```python
from build123d import *

# Parameters (mm, degrees)
SKETCH_1_R          = 2
EXTRUDE_1_DEPTH     = 4
SKETCH_2_R          = 1.5
SKETCH_2_R_2        = 2
EXTRUDE_2_DEPTH     = 4
CUT_EXTRUDE_1_DEPTH = 174.943237868
FILLET_2_R          = 1
FILLET_3_R          = 1


with BuildPart() as part:
    # 草图1 → 凸台-拉伸1 (new body)
    with BuildSketch(Plane(origin=(0, 0, 0), x_dir=(1, 0, 0), z_dir=(0, 1, 0))):
        Polygon((0, 0), (0, -110), (-62.5, -110), (-62.5, -130), (97.5, -130), (97.5, -110), (35, -110), (35, 0), align=None)
        with Locations(Location((5, -5, 0), (0, 0, 270))):
            Circle(SKETCH_1_R, mode=Mode.SUBTRACT)
        with Locations(Location((30, -5, 0), (0, 0, 270))):
            Circle(SKETCH_1_R, mode=Mode.SUBTRACT)
        with Locations(Location((5, -35, 0), (0, 0, 270))):
            Circle(SKETCH_1_R, mode=Mode.SUBTRACT)
        with Locations(Location((30, -35, 0), (0, 0, 270))):
            Circle(SKETCH_1_R, mode=Mode.SUBTRACT)
        with Locations(Location((-52.5, -122.5, 0), (0, 0, 270))):
            Circle(SKETCH_1_R, mode=Mode.SUBTRACT)
        with Locations(Location((-32.5, -122.5, 0), (0, 0, 270))):
            Circle(SKETCH_1_R, mode=Mode.SUBTRACT)
        with Locations(Location((-12.5, -122.5, 0), (0, 0, 270))):
            Circle(SKETCH_1_R, mode=Mode.SUBTRACT)
        with Locations(Location((7.5, -122.5, 0), (0, 0, 270))):
            Circle(SKETCH_1_R, mode=Mode.SUBTRACT)
        with Locations(Location((27.5, -122.5, 0), (0, 0, 270))):
            Circle(SKETCH_1_R, mode=Mode.SUBTRACT)
        with Locations(Location((47.5, -122.5, 0), (0, 0, 270))):
            Circle(SKETCH_1_R, mode=Mode.SUBTRACT)
        with Locations(Location((67.5, -122.5, 0), (0, 0, 270))):
            Circle(SKETCH_1_R, mode=Mode.SUBTRACT)
        with Locations(Location((87.5, -122.5, 0), (0, 0, 270))):
            Circle(SKETCH_1_R, mode=Mode.SUBTRACT)
    extrude(amount=EXTRUDE_1_DEPTH)

    # 草图2 → 凸台-拉伸2 (add)
    # profile 1 of 2: a face of its own
    with BuildSketch(Plane(origin=(0, 4, 0), x_dir=(1, 0, 0), z_dir=(0, 1, 0))):
        Polygon((0, -40), (0, -53), (-26.149225941, -56.891259047), (-32, -65), (-32, -110), (-41, -110), (-41, -70.637206461), (-69.401796613, -110), (-62.5, -110), (-62.5, -130), (-80.5, -130), (-80.5, -110), (-33.599955214, -45), align=None)
        with Locations(Location((-35, -65, 0), (0, 0, 270))):
            Circle(SKETCH_2_R, mode=Mode.SUBTRACT)
        with Locations(Location((-35, -75, 0), (0, 0, 270))):
            Circle(SKETCH_2_R, mode=Mode.SUBTRACT)
        with Locations(Location((-72.5, -122.5, 0), (0, 0, 270))):
            Circle(SKETCH_2_R_2, mode=Mode.SUBTRACT)
    # profile 2 of 2: a face of its own
    with BuildSketch(Plane(origin=(0, 4, 0), x_dir=(1, 0, 0), z_dir=(0, 1, 0))):
        Polygon((67, -65), (67, -110), (76, -110), (76, -70.637206461), (104.401796613, -110), (97.5, -110), (97.5, -130), (115.5, -130), (115.5, -110), (68.599955214, -45), (35, -40), (35, -53), (61.149225941, -56.891259047), align=None)
        with Locations(Location((70, -65, 0), (0, 0, 270))):
            Circle(SKETCH_2_R, mode=Mode.SUBTRACT)
        with Locations(Location((70, -75, 0), (0, 0, 270))):
            Circle(SKETCH_2_R, mode=Mode.SUBTRACT)
        with Locations(Location((107.5, -122.5, 0), (0, 0, 270))):
            Circle(SKETCH_2_R_2, mode=Mode.SUBTRACT)
    extrude(amount=-EXTRUDE_2_DEPTH)

    # 草图3 → 切除-拉伸1 (cut, through all)
    with BuildSketch(Plane(origin=(0, 4, 0), x_dir=(1, 0, 0), z_dir=(0, 1, 0))):
        Polygon((0, -53), (35, -53), (35, -110), (60.5, -110), (60.5, -130), (-25.5, -130), (-25.5, -110), (0, -110), align=None)
    extrude(amount=-CUT_EXTRUDE_1_DEPTH, mode=Mode.SUBTRACT)

    # 圆角2
    fillet_2_edges = [part.edges().sort_by_distance(p)[0] for p in [
        (76, 2, 70.637206461),
        (104.401796613, 2, 110),
        (76, 2, 110),
        (-41, 2, 70.637206461),
        (-41, 2, 110),
        (-69.401796613, 2, 110),
    ]]
    fillet(fillet_2_edges, radius=FILLET_2_R)

    # 圆角3
    fillet_3_edges = [part.edges().sort_by_distance(p)[0] for p in [
        (115.5, 2, 130),
        (115.5, 2, 110),
        (68.599955214, 2, 45),
        (60.5, 2, 110),
        (60.5, 2, 130),
        (-25.5, 2, 130),
        (-25.5, 2, 110),
        (-33.599955214, 2, 45),
        (-80.5, 2, 110),
        (-80.5, 2, 130),
    ]]
    fillet(fillet_3_edges, radius=FILLET_3_R)


solid = part.part
```
The listing builds one solid part. Answer for the finished solid, in the listing's coordinates (mm). A direction names the side the tool comes from. Round coordinates to 2 decimals unless told otherwise and drop trailing zeros. Write each loop counter-clockwise with the first axis right and the second up, starting at its lowest first coordinate (ties: lowest second). Pieces come first, ordered by that corner, then holes. Notation, with made-up numbers: (40.5, 71) -> (68.5, 71) arc R20 cw to (68.5, 89) -> close; hole circle Ø11 at (-1.75, 71.5). An arc over 180 degrees is marked (long way). Use CSV: the item, a comma, the result in double quotes. Start each with the question number.
(1) Consider L1, parallel to X at y = 2.35, z = 5; L2, parallel to Z at x = 66, y = 0.9; L3, parallel to X at y = 1.1, z = 75. Determine where each line is inside the solid, lowest interval first. Write a range as from..to.
(2) Section B-B on z = 5 is taken. Give the vertices of the cut face in (x, y), then the cut area to 3 significant figures.
(3) The mould has two halves that part along Z. Classify faces 1 (the face through (90, 2, 110)), 2 (the face through (28, 2, 5)), 3 (the face through (-53, 2, 130)), 4 (the face through (92.404, 2.028, 77.991)): released by +Z, released by -Z, zero draft, split by the parting line, or undercut.
(4) Section D-D on x = -57.5 is taken. Give the vertices of the cut face in (y, z).
(5) Section A-A on x = 30 is taken. Give the vertices of the cut face in (y, z).
(6) Which of the six approach directions +Z, -Z, +X, -X, +Y, -Y give full straight-line access (tool end or side, diameter ignored) to faces 5 (the face through (35, 2, 20)), 6 (the face through (-57.404, 2.028, 77.991)), 7 (the face through (-25.5, 2, 120)), 8 (the face through (-41, 2, 92))?
(7) Each of these flat-tipped pins is pushed along its axis until it touches: pin 1 (2 mm diameter, centred on x = 55.5, y = 1, fed in from -Z); pin 2 (2 mm diameter, centred on y = 1, z = 30, fed in from -X); pin 3 (1 mm diameter, centred on y = 1, z = 96, fed in from +X). Where does it stop, or does it pass through?
(8) Section C-C on z = 99 is taken. Give the vertices of the cut face in (x, y).
A:
1,L1,"x = 0..3, 7..28, 32..35"
1,L2,"z = 44.61..63.61, 110..121.18, 123.82..130"
1,L3,"x = -55.25..-44.15, -41..-36.5, -33.5..-32, 67..68.5, 71.5..76, 79.15..90.25"
2,outline,"(0, 0) -> (3, 0) -> (3, 4) -> (0, 4) -> close; (7, 0) -> (28, 0) -> (28, 4) -> (7, 4) -> close; (32, 0) -> (35, 0) -> (35, 4) -> (32, 4) -> close"
2,area,"108 mm²"
3,face 1,"undercut"
3,face 2,"undercut"
3,face 3,"released by +Z"
3,face 4,"released by -Z"
4,outline,"(0, 78.12) -> (4, 78.12) -> (4, 93.5) -> (0, 93.5) -> close; (0, 110) -> (4, 110) -> (4, 130) -> (0, 130) -> close"
5,outline,"(0, 0) -> (4, 0) -> (4, 3) -> (0, 3) -> close; (0, 7) -> (4, 7) -> (4, 33) -> (0, 33) -> close; (0, 37) -> (4, 37) -> (4, 53) -> (0, 53) -> close"
6,face 5,"-Z, +X, +Y, -Y"
6,face 6,"-Z, -X, +Y, -Y"
6,face 7,"+Z, +Y, -Y"
6,face 8,"+Y, -Y"
7,pin 1,"stops at z = 42.9"
7,pin 2,"stops at x = 0"
7,pin 3,"stops at x = 105.76"
8,outline,"(-72.56, 0) -> (-61.46, 0) -> (-61.46, 4) -> (-72.56, 4) -> close; (-41, 0) -> (-32, 0) -> (-32, 4) -> (-41, 4) -> close; (67, 0) -> (76, 0) -> (76, 4) -> (67, 4) -> close; (96.46, 0) -> (107.56, 0) -> (107.56, 4) -> (96.46, 4) -> close"
